from build123d import *

# Parameters (mm, degrees)
SKETCH1_W                   = 150
SKETCH1_H                   = 150.9
BOSS_EXTRUDE1_DEPTH         = 10
SKETCH2_R                   = 9.075
SKETCH2_W                   = 19.6
SKETCH2_H                   = 12.7
SKETCH2_W_2                 = 19.05
SKETCH2_H_2                 = 11.7
SKETCH2_W_3                 = 28
SKETCH2_H_3                 = 28
CUT_EXTRUDE1_DEPTH          = 10
FILLET1_R                   = 8
FILLET2_R                   = 3
SKETCH5_R                   = 4.075
CUT_EXTRUDE4_DEPTH          = 10
MIRROR3_COPY_1_SKETCH_R     = 4.075
MIRROR3_COPY_1_DEPTH        = 10
FILLET6_R                   = 3
CUT_EXTRUDE6_DEPTH          = 11
LPATTERN3_COUNT             = 2
LPATTERN3_PITCH             = 120
SKETCH9_R                   = 6.075
SKETCH9_R_2                 = 4.075
BOSS_EXTRUDE2_DEPTH         = 8
LPATTERN4_COUNT             = 2
LPATTERN4_PITCH             = 134
LPATTERN5_COUNT             = 2
LPATTERN5_PITCH             = 134
LPATTERN5_COPY_1_SKETCH_R   = 6.075
LPATTERN5_COPY_1_SKETCH_R_2 = 4.075
LPATTERN5_COPY_1_DEPTH      = 8
BOSS_EXTRUDE4_DEPTH         = 8
SKETCH12_W                  = 19.1
SKETCH12_H                  = 16.2
CUT_EXTRUDE7_DEPTH          = 2.07


with BuildPart() as part:
    # Sketch1 → Boss-Extrude1 (new body)
    with BuildSketch(Plane(origin=(0, 0, 0), x_dir=(1, 0, 0), z_dir=(0, 1, 0))):
        Rectangle(SKETCH1_W, SKETCH1_H)
    extrude(amount=BOSS_EXTRUDE1_DEPTH)

    # Sketch2 → Cut-Extrude1 (cut)
    with BuildSketch(Plane(origin=(0, 10, 0), x_dir=(1, 0, 0), z_dir=(0, 1, 0))):
        with Locations((-35.2, 56.75)):
            Circle(SKETCH2_R)
        with Locations((0, 56.75)):
            Circle(SKETCH2_R)
        with Locations((35.2, 56.75)):
            Circle(SKETCH2_R)
        with Locations((-35.2, 18.6)):
            Circle(SKETCH2_R)
        with Locations((0, 18.6)):
            Circle(SKETCH2_R)
        with Locations((0, -16.825)):
            Rectangle(SKETCH2_W, SKETCH2_H)
        with Locations((-35.2, -16.825)):
            Rectangle(SKETCH2_W, SKETCH2_H)
        with Locations((35.2, -16.825)):
            Rectangle(SKETCH2_W, SKETCH2_H)
        with Locations((-35.2, -49.025)):
            Rectangle(SKETCH2_W_2, SKETCH2_H_2)
        with Locations((0, -49.025)):
            Rectangle(SKETCH2_W_2, SKETCH2_H_2)
        with Locations((35.2, -49.025)):
            Rectangle(SKETCH2_W_2, SKETCH2_H_2)
        with Locations((35.2, 18.6)):
            Rectangle(SKETCH2_W_3, SKETCH2_H_3)
    extrude(amount=-CUT_EXTRUDE1_DEPTH, mode=Mode.SUBTRACT)

    # Fillet1
    fillet1_edges = [part.edges().sort_by_distance(p)[0] for p in [
        (75, 5, 75.45),
        (-75, 5, 75.45),
        (-75, 5, -75.45),
        (75, 5, -75.45),
    ]]
    fillet(fillet1_edges, radius=FILLET1_R)

    # Fillet2
    fillet2_edges = [part.edges().sort_by_distance(p)[0] for p in [
        (25.4, 5, 23.175),
        (25.4, 5, 10.475),
        (45, 5, 10.475),
        (45, 5, 23.175),
        (-44.725, 5, 54.875),
        (-44.725, 5, 43.175),
        (-25.675, 5, 43.175),
        (-25.675, 5, 54.875),
        (-9.525, 5, 54.875),
        (-9.525, 5, 43.175),
        (9.525, 5, 43.175),
        (9.525, 5, 54.875),
        (25.675, 5, 54.875),
        (25.675, 5, 43.175),
        (44.725, 5, 43.175),
        (44.725, 5, 54.875),
        (-9.8, 5, 23.175),
        (-9.8, 5, 10.475),
        (9.8, 5, 10.475),
        (9.8, 5, 23.175),
        (-45, 5, 23.175),
        (-45, 5, 10.475),
        (-25.4, 5, 10.475),
        (-25.4, 5, 23.175),
    ]]
    fillet(fillet2_edges, radius=FILLET2_R)

    # Sketch5 → Cut-Extrude4 (cut)
    with BuildSketch(Plane(origin=(0, 10, 0), x_dir=(1, 0, 0), z_dir=(0, 1, 0))):
        with Locations((-67, 67.45)):
            Circle(SKETCH5_R)
    cut_extrude4 = extrude(amount=-CUT_EXTRUDE4_DEPTH, mode=Mode.SUBTRACT)

    # Mirror1: Cut-Extrude4 across plane
    add(cut_extrude4.mirror(Plane.XY), mode=Mode.SUBTRACT)

    # Mirror3: Cut-Extrude4 across plane
    add(cut_extrude4.mirror(Plane(origin=(0, 0, 0), x_dir=(0, 0, 1), z_dir=(1, 0, 0))), mode=Mode.SUBTRACT)

    # Mirror3 copy 1 sketch → Mirror3 copy 1 (cut)
    with BuildSketch(Plane(origin=(0, 10, 0), x_dir=(-1, 0, 0), z_dir=(0, 1, 0))):
        with Locations((-67, 67.45)):
            Circle(MIRROR3_COPY_1_SKETCH_R)
    extrude(amount=-MIRROR3_COPY_1_DEPTH, mode=Mode.SUBTRACT)

    # Fillet6
    fillet6_edges = [part.edges().sort_by_distance(p)[0] for p in [
        (21.2, 5, -32.6),
        (49.2, 5, -32.6),
    ]]
    fillet(fillet6_edges, radius=FILLET6_R)

    # Sketch7 → Cut-Extrude6 (cut, through all)
    with BuildSketch(Plane(origin=(0, 10, 0), x_dir=(1, 0, 0), z_dir=(0, 1, 0))):
        with BuildLine():
            Line((60.272487235, 48.384614922), (60.272487235, -35.499184585))
            ThreePointArc((60.272487235, -35.499184585), (58.278399823, -37.493271997), (56.284312411, -35.499184585))
            Line((56.284312411, -35.499184585), (56.284312411, 48.384614922))
            ThreePointArc((56.284312411, 48.384614922), (58.278399823, 50.378702334), (60.272487235, 48.384614922))
        make_face()
        with BuildLine():
            Line((66.651655516, 32.551344452), (66.651655516, -51.076821304))
            ThreePointArc((66.651655516, -51.076821304), (64.83996028, -52.88851654), (63.028265044, -51.076821304))
            Line((63.028265044, -51.076821304), (63.028265044, 32.551344452))
            ThreePointArc((63.028265044, 32.551344452), (64.83996028, 34.363039688), (66.651655516, 32.551344452))
        make_face()
    cut_extrude6 = extrude(amount=-CUT_EXTRUDE6_DEPTH, mode=Mode.SUBTRACT)

    # LPattern3: Cut-Extrude6 ×2
    with Locations(*[(-i * LPATTERN3_PITCH, 0, 0) for i in range(1, LPATTERN3_COUNT)]):
        add(cut_extrude6, mode=Mode.SUBTRACT)

    # Sketch9 → Boss-Extrude2 (add)
    with BuildSketch(Plane(origin=(0, 10, 0), x_dir=(1, 0, 0), z_dir=(0, 1, 0))):
        with Locations((-67, 67.45)):
            Circle(SKETCH9_R)
        with Locations((-67, 67.45)):
            Circle(SKETCH9_R_2, mode=Mode.SUBTRACT)
    boss_extrude2 = extrude(amount=BOSS_EXTRUDE2_DEPTH)

    # LPattern4: Boss-Extrude2 ×2
    with Locations(*[(i * LPATTERN4_PITCH, 0, 0) for i in range(1, LPATTERN4_COUNT)]):
        add(boss_extrude2)

    # LPattern5: Boss-Extrude2 ×2
    with Locations(*[(0, 0, i * LPATTERN5_PITCH) for i in range(1, LPATTERN5_COUNT)]):
        add(boss_extrude2)

    # LPattern5 copy 1 sketch → LPattern5 copy 1 (add)
    with BuildSketch(Plane(origin=(134, 10, 134), x_dir=(1, 0, 0), z_dir=(0, 1, 0))):
        with Locations((-67, 67.45)):
            Circle(LPATTERN5_COPY_1_SKETCH_R)
        with Locations((-67, 67.45)):
            Circle(LPATTERN5_COPY_1_SKETCH_R_2, mode=Mode.SUBTRACT)
    extrude(amount=LPATTERN5_COPY_1_DEPTH)

    # Sketch10 → Boss-Extrude4 (add)
    with BuildSketch(Plane(origin=(0, 10, 0), x_dir=(1, 0, 0), z_dir=(0, 1, 0))):
        with BuildLine():
            Line((-67, 75.45), (67, 75.45))
            ThreePointArc((67, 75.45), (72.656854249, 73.106854249), (75, 67.45))
            Line((75, 67.45), (75, -67.45))
            ThreePointArc((75, -67.45), (72.656854249, -73.106854249), (67, -75.45))
            Line((67, -75.45), (-67, -75.45))
            ThreePointArc((-67, -75.45), (-72.656854249, -73.106854249), (-75, -67.45))
            Line((-75, -67.45), (-75, 67.45))
            ThreePointArc((-75, 67.45), (-72.656854249, 73.106854249), (-67, 75.45))
        make_face()
        with BuildLine():
            Line((-67, 73.525), (67, 73.525))
            ThreePointArc((67, 73.525), (71.295673696, 71.745673696), (73.075, 67.45))
            Line((73.075, 67.45), (73.075, -66.55))
            ThreePointArc((73.075, -66.55), (71.295673696, -70.845673696), (67, -72.625))
            Line((67, -72.625), (-67, -72.625))
            ThreePointArc((-67, -72.625), (-71.295673696, -70.845673696), (-73.075, -66.55))
            Line((-73.075, -66.55), (-73.075, 67.45))
            ThreePointArc((-73.075, 67.45), (-71.295673696, 71.745673696), (-67, 73.525))
        make_face(mode=Mode.SUBTRACT)
    extrude(amount=BOSS_EXTRUDE4_DEPTH)

    # Sketch12 → Cut-Extrude7 (cut)
    with BuildSketch(Plane(origin=(0, 10, 0), x_dir=(1, 0, 0), z_dir=(0, 1, 0))):
        with Locations((0.98628476, 0.329027808)):
            Rectangle(SKETCH12_W, SKETCH12_H)
    extrude(amount=-CUT_EXTRUDE7_DEPTH, mode=Mode.SUBTRACT)


solid = part.part
CAD build for the part. Positions are in the model's coordinates, mm. A direction names the side the tool comes from. Round coordinates to 2 decimals unless told otherwise and drop trailing zeros. Loops run counter-clockwise (first coordinate to the right, second up) from the corner with the lowest first, then second, coordinate; pieces in that order, holes last.
(1) Cut at A-A (x = 35.2). Give the cut face in (y, z) (3 decimals), plus the area to 4 significant figures.
(2) Cut at B-B (y = 16.25). Give the cut face in (x, z) (3 decimals), plus the area to 3 significant figures.
(3) Wall check: line 1 along X through (y, z) = (4, 9.5); line 2 along Z through (x, y) = (0, 5.5) (3 decimals); line 3 along X through (y, z) = (2.75, -39). Give the ranges that are in metal, low to high.
(4) Drop flat-ended pins along their axis: pin 1 (1.5 mm diameter, centred on x = -2.5, z = -2.5, fed in from +Y); pin 2 (6 mm diameter, centred on x = 50.5, z = 36, fed in from +Y). Give the stop position or say it passes through.
(5) Cut at D-D (z = -18.6). State how many separate pieces and enclosed holes the cut face has, plus the area to 3 significant figures.
(6) Two-plate mould, pull along X, no slides. Class faces 1 (the flat face through (-1, 0, -1)), 2 (the flat face through (35, 5, -32.6)), 3 (the cylindrical face through (65.12, 5.07, 63.835)): +X half, -X half, draft (parallel to the pull), parting line (faces both ways), or undercut.
(7) Cut at C-C (z = -56.75). Give the cut face in (x, y) (3 decimals), plus the area to 3 significant figures.
(8) Which spindle directions (+Z, -Z, +X, -X, +Y, -Y) get a long thin tool onto all of the face, cutting with end or side? Do faces 4 (the flat face through (67, 10, 71)), 5 (the flat face through (67, 10, 63)), 6 (the flat face through (0, 5, 10.475)). Say none if no direction does.
Findings below:
1. outline: (0, -75.45) - (18, -75.45) - (18, -73.525) - (10, -73.525) - (10, -65.825) - (0, -65.825) - close; (0, -47.675) - (10, -47.675) - (10, -32.6) - (0, -32.6) - close; (0, -4.6) - (10, -4.6) - (10, 10.475) - (0, 10.475) - close; (0, 23.175) - (10, 23.175) - (10, 43.175) - (0, 43.175) - close; (0, 54.875) - (10, 54.875) - (10, 72.625) - (18, 72.625) - (18, 75.45) - (0, 75.45) - close
1. area: 841.5 mm2
2. outline: (-75, -67.45) arc R8 ccw to (-67, -75.45) - (67, -75.45) arc R8 ccw to (75, -67.45) - (75, 67.45) arc R8 ccw to (67, 75.45) - (-67, 75.45) arc R8 ccw to (-75, 67.45) - close; hole (-73.075, -67.45) arc R6.075 cw (long way) to (-67, -73.525) - (67, -73.525) arc R6.075 cw (long way) to (73.075, -67.45) - (73.075, 66.55) arc R6.075 cw (long way) to (67, 72.625) - (-67, 72.625) arc R6.075 cw (long way) to (-73.075, 66.55) - close; hole circle Ø8.15 at (-67, -67.45); hole circle Ø8.15 at (-67, 66.55); hole circle Ø8.15 at (67, -67.45); hole circle Ø8.15 at (67, 66.55)
2. area: 1,510 mm2
3. line 1: x = -75 to -63.72, -59.73 to -56.97, -53.35 to 56.28, 60.27 to 63.03, 66.65 to 75
3. line 2: z = -75.45 to -65.825, -47.675 to -27.675, -9.525 to 10.475, 23.175 to 43.175, 54.875 to 75.45
3. line 3: x = -75 to -63.72, -59.73 to 56.28, 60.27 to 75
4. pin 1: stops at y = 7.93
4. pin 2: stops at y = 10
5. separate pieces: 8
5. enclosed holes: 0
5. area: 736 mm2
6. face 1: draft
6. face 2: undercut
6. face 3: undercut
7. outline: (-75, 0) - (-44.275, 0) - (-44.275, 10) - (-73.075, 10) - (-73.075, 18) - (-75, 18) - close; (-26.125, 0) - (-9.075, 0) - (-9.075, 10) - (-26.125, 10) - close; (9.075, 0) - (26.125, 0) - (26.125, 10) - (9.075, 10) - close; (44.275, 0) - (75, 0) - (75, 18) - (73.075, 18) - (73.075, 10) - (44.275, 10) - close
7. area: 986 mm2
8. face 4: -Y
8. face 5: +Y
8. face 6: +Y, -Y
